Geometry check sheet. Reference: drawing and pictorial views, mm from the part's lowest x, y, z. A direction names the side the tool comes from. Give positions to 0.01 mm unless a question says otherwise; leave off trailing zeros. Order: outer loops, then holes, each group sorted by start corner. A loop starts at its lowest first (then second) coordinate and runs counter-clockwise, first axis right, second up.
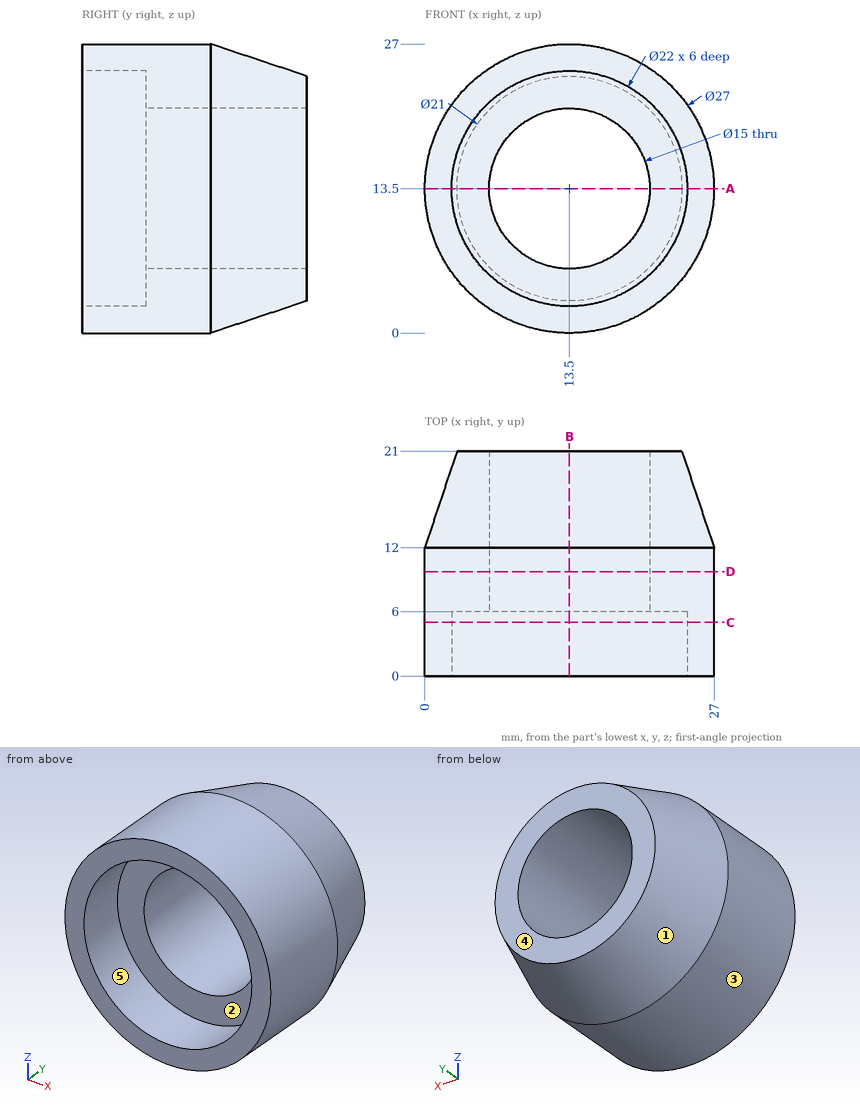
1) Set-up check for the marked faces 1 and 2: record each of +Z, -Z, +X, -X, +Y, -Y from which the full face is reachable in a straight line by a thin tool's end or side.
Recorded:
face 1: +Y
face 2: -Y
2) Section check C-C, the plane y = 5. Record the cut outline in (x, z).
Recorded:
outline: circle Ø27 at (13.5, 13.5); hole circle Ø22 at (13.5, 13.5)
3) Draft check along Z on the marked faces 3, 4 and 5. Enter one of: +Z half, -Z half, draft (parallel to the pull), parting line (faces both ways), or undercut.
Recorded:
face 3: parting line
face 4: draft
face 5: undercut
4) Section check A-A, the plane z = 13.5. Record the cut outline in (x, y), then the cut area to 3 significant figures.
Recorded:
outline: (0, 0) - (2.5, 0) - (2.5, 6) - (6, 6) - (6, 21) - (3, 21) - (0, 12) - close; (21, 6) - (24.5, 6) - (24.5, 0) - (27, 0) - (27, 12) - (24, 21) - (21, 21) - close
area: 183 mm2
5) Material ranges on L1, parallel to Z at x = 13.5, y = 4.55; L2, parallel to Z at x = 13.5, y = 11, recorded low to high.
Recorded:
L1: z = 0 to 2.5, 24.5 to 27
L2: z = 0 to 6, 21 to 27
6) Section check B-B, the plane x = 13.5. Record the cut outline in (y, z), then the cut area to 3 significant figures.
Recorded:
outline: (0, 0) - (12, 0) - (21, 3) - (21, 6) - (6, 6) - (6, 2.5) - (0, 2.5) - close; (0, 24.5) - (6, 24.5) - (6, 21) - (21, 21) - (21, 24) - (12, 27) - (0, 27) - close
area: 183 mm2
7) Depth check by flat-ended pin: pin 1 Ø4 at (y, z) = (6.5, 6.5) entering from +X; pin 2 Ø6 at (y, z) = (14.5, 5.5) entering from -X; pin 3 Ø4 at (x, y) = (18, 10) entering from -Z; pin 4 Ø10 at (x, z) = (2.5, 20) entering from -Y. Enter the tip coordinate at first touch or a pass-through.
Recorded:
pin 1: stops at x = 26.04
pin 2: stops at x = 1.47
pin 3: stops at z = 0.23
pin 4: stops at y = 0
8) Section check D-D, the plane y = 9.75. Record the cut outline in (x, z).
Recorded:
outline: circle Ø27 at (13.5, 13.5); hole circle Ø15 at (13.5, 13.5)
